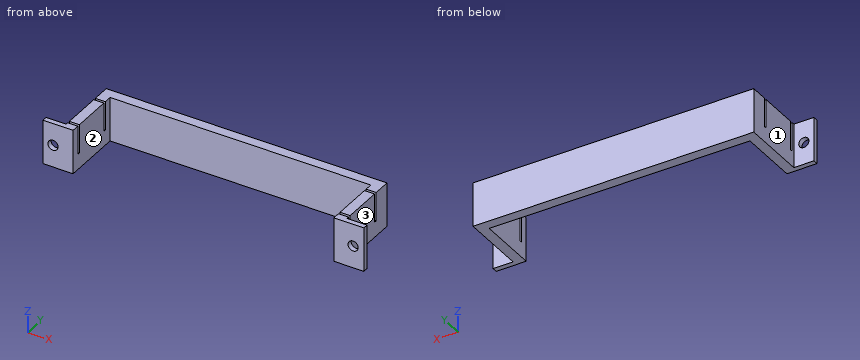
```python
from build123d import *

# Parameters (mm, degrees)
SKETCH1_W           = 160
SKETCH1_H           = 22
BOSS_EXTRUDE1_DEPTH = 35
SKETCH4_W           = 130
SKETCH4_H           = 30
CUT_EXTRUDE3_DEPTH  = 23
SKETCH5_W           = 10
SKETCH5_H           = 32.46
CUT_EXTRUDE4_DEPTH  = 23
SKETCH7_W           = 14.38
SKETCH7_H           = 1.27
CUT_EXTRUDE5_DEPTH  = 151
SKETCH8_R           = 2.54
CUT_EXTRUDE6_DEPTH  = 3.54


with BuildPart() as part:
    # Sketch1 → Boss-Extrude1 (new body)
    with BuildSketch(Plane(origin=(0, 0, 0), x_dir=(1, 0, 0), z_dir=(0, 1, 0))):
        with Locations((80, 11)):
            Rectangle(SKETCH1_W, SKETCH1_H)
    extrude(amount=BOSS_EXTRUDE1_DEPTH)

    # Sketch4 → Cut-Extrude3 (cut, through all)
    with BuildSketch(Plane.XY):
        with Locations((80, 15)):
            Rectangle(SKETCH4_W, SKETCH4_H)
    extrude(amount=-CUT_EXTRUDE3_DEPTH, mode=Mode.SUBTRACT)

    # Sketch5 → Cut-Extrude4 (cut, through all)
    with BuildSketch(Plane.XY):
        with Locations((5, 18.77)):
            Rectangle(SKETCH5_W, SKETCH5_H)
        with Locations((155, 18.77)):
            Rectangle(SKETCH5_W, SKETCH5_H)
    extrude(amount=-CUT_EXTRUDE4_DEPTH, mode=Mode.SUBTRACT)

    # Sketch7 → Cut-Extrude5 (cut, through all)
    with BuildSketch(Plane.ZY.offset(-10)):
        with Locations((-7.19, 4.445)):
            Rectangle(SKETCH7_W, SKETCH7_H)
        with Locations((-7.19, 25.555)):
            Rectangle(SKETCH7_W, SKETCH7_H)
    extrude(amount=-CUT_EXTRUDE5_DEPTH, mode=Mode.SUBTRACT)

    # Sketch8 → Cut-Extrude6 (cut, through all)
    with BuildSketch(Plane(origin=(0, 2.54, 0), x_dir=(1, 0, 0), z_dir=(0, 1, 0))):
        with Locations((154.621372276, 11)):
            Circle(SKETCH8_R)
        with Locations((5, 11)):
            Circle(SKETCH8_R)
    extrude(amount=-CUT_EXTRUDE6_DEPTH, mode=Mode.SUBTRACT)


solid = part.part
```
Can you work these out from the model? Positions are in its coordinate system, mm. Face numbers are marked on the shaded views. A direction names the side the tool comes from. Coordinates: 2 decimals unless noted, no trailing zeros. Loops run counter-clockwise (first coordinate to the right, second up) from the corner with the lowest first, then second, coordinate; pieces in that order, holes last.
1) Imagine slicing it at A-A on x = 5. List the corners of the cut face in (y, z) for me.
2) Imagine slicing it at D-D on z = -17. List the corners of the cut face in (x, y) for me.
3) Which directions (+Z, -Z, +X, -X, +Y, -Y) give clear straight access to the entire face, cutting with the end or side of a thin tool? Please do the marked faces 1, 2 and 3.
4) Imagine slicing it at C-C on z = -2.25. List the corners of the cut face in (x, y) for me.
5) Imagine slicing it at B-B on y = 18. List the corners of the cut face in (x, z) for me.
6) I need wall thicknesses on probe 1 along X at (y, z) = (1.1, -11); probe 2 along X at (y, z) = (17, -3.25); probe 3 along Z at (x, y) = (5, 1). Which ranges of each line are inside material? Lowest first, please.
7) For pin 1 (11 mm diameter, centred on y = 12.5, z = -16.5, fed in from +X); pin 2 (1.5 mm diameter, centred on y = 27.5, z = -6, fed in from -X); pin 3 (0.6 mm diameter, centred on x = 148, y = 25.5, fed in from +Z), each with a flat end and sliding along its axis, tell me the tip position at first contact or that it passes through.
Completed:
1. outline: (0, -22) - (2.54, -22) - (2.54, -13.54) - (0, -13.54) - close; (0, -8.46) - (2.54, -8.46) - (2.54, 0) - (0, 0) - close
2. outline: (0, 0) - (15, 0) - (15, 30) - (145, 30) - (145, 0) - (160, 0) - (160, 2.54) - (150, 2.54) - (150, 35) - (10, 35) - (10, 2.54) - (0, 2.54) - close
3. face 1: +Z, -Z, -X, +Y
3. face 2: +Z, -Z, -Y
3. face 3: +Z, -Z, +X, +Y
4. outline: (0, 0) - (15, 0) - (15, 3.81) - (10, 3.81) - (10, 2.54) - (0, 2.54) - close; (10, 5.08) - (15, 5.08) - (15, 24.92) - (10, 24.92) - close; (10, 26.19) - (15, 26.19) - (15, 30) - (145, 30) - (145, 26.19) - (150, 26.19) - (150, 35) - (10, 35) - close; (145, 0) - (160, 0) - (160, 2.54) - (150, 2.54) - (150, 3.81) - (145, 3.81) - close; (145, 5.08) - (150, 5.08) - (150, 24.92) - (145, 24.92) - close
5. outline: (10, -22) - (15, -22) - (15, 0) - (10, 0) - close; (145, -22) - (150, -22) - (150, 0) - (145, 0) - close
6. probe 1: x = 0 to 2.46, 7.54 to 15, 145 to 152.08, 157.16 to 160
6. probe 2: x = 10 to 15, 145 to 150
6. probe 3: z = -22 to -13.54, -8.46 to 0
7. pin 1: stops at x = 150
7. pin 2: stops at x = 10
7. pin 3: stops at z = -14.38
